from build123d import *

# Parameters (mm, degrees)
F1_DEPTH = 1
F3_DEPTH = 0.05
F4_W     = 3.2
F4_H     = 5
F5_DEPTH = 0.9
F6_R     = 0.25


with BuildPart() as f1:
    # F0 (on Front) → F1 (new body)
    with BuildSketch(Plane.XZ):
        Polygon((0, 0.35), (0, 0), (16, 0), (16, 0.35), (15, 0.35), (15, 1.65), (16, 1.65), (16, 2.35), (15, 2.35), (15, 3.65), (16, 3.65), (16, 4.35), (15, 4.35), (15, 5.65), (16, 5.65), (16, 6.35), (15, 6.35), (15, 7.65), (16, 7.65), (16, 8.35), (15, 8.35), (15, 9.65), (16, 9.65), (16, 10.35), (15, 10.35), (15, 11.65), (16, 11.65), (16, 12.35), (15, 12.35), (15, 13.65), (16, 13.65), (16, 14.35), (15, 14.35), (15, 15.65), (16, 15.65), (16, 16), (0, 16), (0, 15.65), (1, 15.65), (1, 14.35), (0, 14.35), (0, 13.65), (1, 13.65), (1, 12.35), (0, 12.35), (0, 11.65), (1, 11.65), (1, 10.35), (0, 10.35), (0, 9.65), (1, 9.65), (1, 8.35), (0, 8.35), (0, 7.65), (1, 7.65), (1, 6.35), (0, 6.35), (0, 5.65), (1, 5.65), (1, 4.35), (0, 4.35), (0, 3.65), (1, 3.65), (1, 2.35), (0, 2.35), (0, 1.65), (1, 1.65), (1, 0.35), align=None)
        with BuildLine():
            ThreePointArc((0, 13.65), (0.380511, 13), (0, 12.35))
            Line((0, 12.35), (1, 12.35))
            Line((1, 12.35), (1, 13.65))
            Line((1, 13.65), (0, 13.65))
        make_face()
        with BuildLine():
            ThreePointArc((0, 11.65), (0.380511, 11), (0, 10.35))
            Line((0, 10.35), (1, 10.35))
            Line((1, 10.35), (1, 11.65))
            Line((1, 11.65), (0, 11.65))
        make_face()
        with BuildLine():
            ThreePointArc((0, 9.65), (0.380511, 9), (0, 8.35))
            Line((0, 8.35), (1, 8.35))
            Line((1, 8.35), (1, 9.65))
            Line((1, 9.65), (0, 9.65))
        make_face()
        with BuildLine():
            ThreePointArc((0, 7.65), (0.380511, 7), (0, 6.35))
            Line((0, 6.35), (1, 6.35))
            Line((1, 6.35), (1, 7.65))
            Line((1, 7.65), (0, 7.65))
        make_face()
        with BuildLine():
            ThreePointArc((0, 5.65), (0.380511, 5), (0, 4.35))
            Line((0, 4.35), (1, 4.35))
            Line((1, 4.35), (1, 5.65))
            Line((1, 5.65), (0, 5.65))
        make_face()
        with BuildLine():
            ThreePointArc((0, 3.65), (0.380511, 3), (0, 2.35))
            Line((0, 2.35), (1, 2.35))
            Line((1, 2.35), (1, 3.65))
            Line((1, 3.65), (0, 3.65))
        make_face()
        with BuildLine():
            ThreePointArc((0, 1.65), (0.380511, 1), (0, 0.35))
            Line((0, 0.35), (1, 0.35))
            Line((1, 0.35), (1, 1.65))
            Line((1, 1.65), (0, 1.65))
        make_face()
        with BuildLine():
            Line((15, 4.35), (16, 4.35))
            ThreePointArc((16, 4.35), (15.619489, 5), (16, 5.65))
            Line((16, 5.65), (15, 5.65))
            Line((15, 5.65), (15, 4.35))
        make_face()
        with BuildLine():
            Line((15, 6.35), (16, 6.35))
            ThreePointArc((16, 6.35), (15.619489, 7), (16, 7.65))
            Line((16, 7.65), (15, 7.65))
            Line((15, 7.65), (15, 6.35))
        make_face()
        with BuildLine():
            Line((15, 8.35), (16, 8.35))
            ThreePointArc((16, 8.35), (15.619489, 9), (16, 9.65))
            Line((16, 9.65), (15, 9.65))
            Line((15, 9.65), (15, 8.35))
        make_face()
        with BuildLine():
            Line((15, 10.35), (16, 10.35))
            ThreePointArc((16, 10.35), (15.619489, 11), (16, 11.65))
            Line((16, 11.65), (15, 11.65))
            Line((15, 11.65), (15, 10.35))
        make_face()
        with BuildLine():
            Line((15, 12.35), (16, 12.35))
            ThreePointArc((16, 12.35), (15.619489, 13), (16, 13.65))
            Line((16, 13.65), (15, 13.65))
            Line((15, 13.65), (15, 12.35))
        make_face()
        with BuildLine():
            Line((15, 14.35), (16, 14.35))
            ThreePointArc((16, 14.35), (15.619489, 15), (16, 15.65))
            Line((16, 15.65), (15, 15.65))
            Line((15, 15.65), (15, 14.35))
        make_face()
        with BuildLine():
            Line((15, 2.35), (16, 2.35))
            ThreePointArc((16, 2.35), (15.619489, 3), (16, 3.65))
            Line((16, 3.65), (15, 3.65))
            Line((15, 3.65), (15, 2.35))
        make_face()
        with BuildLine():
            Line((15, 0.35), (16, 0.35))
            ThreePointArc((16, 0.35), (15.619489, 1), (16, 1.65))
            Line((16, 1.65), (15, 1.65))
            Line((15, 1.65), (15, 0.35))
        make_face()
        with BuildLine():
            ThreePointArc((0, 15.65), (0.380511, 15), (0, 14.35))
            Line((0, 14.35), (1, 14.35))
            Line((1, 14.35), (1, 15.65))
            Line((1, 15.65), (0, 15.65))
        make_face()
    extrude(amount=F1_DEPTH)

    # F2 (on face) → F3 (join)
    with BuildSketch(Plane.XZ.offset(1)):
        with BuildLine():
            ThreePointArc((16, 14.35), (15.619489, 15), (16, 15.65))
            Line((16, 15.65), (15, 15.65))
            Line((15, 15.65), (15, 14.35))
            Line((15, 14.35), (16, 14.35))
        make_face()
        with BuildLine():
            ThreePointArc((16, 12.35), (15.619493, 12.997842), (15.996242, 13.647876))
            Line((15.996242, 13.647876), (15, 13.647876))
            Line((15, 13.647876), (15, 12.347876))
            Line((15, 12.347876), (16, 12.347876))
            Line((16, 12.347876), (16, 12.35))
        make_face()
        with BuildLine():
            ThreePointArc((16, 10.35), (15.619502, 10.995706), (15.992535, 11.645752))
            Line((15.992535, 11.645752), (15, 11.645752))
            Line((15, 11.645752), (15, 10.345752))
            Line((15, 10.345752), (16, 10.345752))
            Line((16, 10.345752), (16, 10.35))
        make_face()
        with BuildLine():
            ThreePointArc((16, 8.35), (15.619517, 8.99359), (15.988876, 9.643628))
            Line((15.988876, 9.643628), (15, 9.643628))
            Line((15, 9.643628), (15, 8.343628))
            Line((15, 8.343628), (16, 8.343628))
            Line((16, 8.343628), (16, 8.35))
        make_face()
        with BuildLine():
            ThreePointArc((16, 6.35), (15.619538, 6.991495), (15.985264, 7.641505))
            Line((15.985264, 7.641505), (15, 7.641505))
            Line((15, 7.641505), (15, 6.341505))
            Line((15, 6.341505), (16, 6.341505))
            Line((16, 6.341505), (16, 6.35))
        make_face()
        with BuildLine():
            ThreePointArc((16, 4.35), (15.619565, 4.98942), (15.981698, 5.639381))
            Line((15.981698, 5.639381), (15, 5.639381))
            Line((15, 5.639381), (15, 4.339381))
            Line((15, 4.339381), (16, 4.339381))
            Line((16, 4.339381), (16, 4.35))
        make_face()
        with BuildLine():
            ThreePointArc((16, 2.35), (15.619597, 2.987364), (15.978177, 3.637257))
            Line((15.978177, 3.637257), (15, 3.637257))
            Line((15, 3.637257), (15, 2.337257))
            Line((15, 2.337257), (16, 2.337257))
            Line((16, 2.337257), (16, 2.35))
        make_face()
        with BuildLine():
            ThreePointArc((16, 0.35), (15.619634, 0.985327), (15.974699, 1.635133))
            Line((15.974699, 1.635133), (15, 1.635133))
            Line((15, 1.635133), (15, 0.335133))
            Line((15, 0.335133), (16, 0.335133))
            Line((16, 0.335133), (16, 0.35))
        make_face()
        with BuildLine():
            Line((1, 1.635133), (0.025301, 1.635133))
            ThreePointArc((0.025301, 1.635133), (0.380366, 0.985327), (0, 0.35))
            Line((0, 0.35), (0, 0.335133))
            Line((0, 0.335133), (1, 0.335133))
            Line((1, 0.335133), (1, 1.635133))
        make_face()
        with BuildLine():
            Line((1, 3.637257), (0.021823, 3.637257))
            ThreePointArc((0.021823, 3.637257), (0.380403, 2.987364), (0, 2.35))
            Line((0, 2.35), (0, 2.337257))
            Line((0, 2.337257), (1, 2.337257))
            Line((1, 2.337257), (1, 3.637257))
        make_face()
        with BuildLine():
            Line((1, 5.639381), (0.018302, 5.639381))
            ThreePointArc((0.018302, 5.639381), (0.380435, 4.98942), (0, 4.35))
            Line((0, 4.35), (0, 4.339381))
            Line((0, 4.339381), (1, 4.339381))
            Line((1, 4.339381), (1, 5.639381))
        make_face()
        with BuildLine():
            Line((1, 7.641505), (0.014736, 7.641505))
            ThreePointArc((0.014736, 7.641505), (0.380462, 6.991495), (0, 6.35))
            Line((0, 6.35), (0, 6.341505))
            Line((0, 6.341505), (1, 6.341505))
            Line((1, 6.341505), (1, 7.641505))
        make_face()
        with BuildLine():
            Line((1, 9.643628), (0.011124, 9.643628))
            ThreePointArc((0.011124, 9.643628), (0.380483, 8.99359), (0, 8.35))
            Line((0, 8.35), (0, 8.343628))
            Line((0, 8.343628), (1, 8.343628))
            Line((1, 8.343628), (1, 9.643628))
        make_face()
        with BuildLine():
            Line((1, 11.645752), (0.007465, 11.645752))
            ThreePointArc((0.007465, 11.645752), (0.380498, 10.995706), (0, 10.35))
            Line((0, 10.35), (0, 10.345752))
            Line((0, 10.345752), (1, 10.345752))
            Line((1, 10.345752), (1, 11.645752))
        make_face()
        with BuildLine():
            Line((1, 13.647876), (0.003758, 13.647876))
            ThreePointArc((0.003758, 13.647876), (0.380507, 12.997842), (0, 12.35))
            Line((0, 12.35), (0, 12.347876))
            Line((0, 12.347876), (1, 12.347876))
            Line((1, 12.347876), (1, 13.647876))
        make_face()
        with BuildLine():
            Line((1, 15.65), (0, 15.65))
            ThreePointArc((0, 15.65), (0.380511, 15), (0, 14.35))
            Line((0, 14.35), (1, 14.35))
            Line((1, 14.35), (1, 15.65))
        make_face()
    extrude(amount=F3_DEPTH)

    # F4 (on face) → F5 (join)
    with BuildSketch(Plane.XZ.offset(1)):
        with Locations((11.804315, 7.033254)):
            Rectangle(F4_W, F4_H)
    extrude(amount=F5_DEPTH)

    # F6
    f6_edges = [f1.edges().sort_by_distance(p)[0] for p in [
        (10.204315, -1.45, 4.533254),
        (13.404315, -1.45, 4.533254),
        (10.204315, -1.45, 9.533254),
        (13.404315, -1.45, 9.533254),
    ]]
    fillet(f6_edges, radius=F6_R)


solid = f1.part
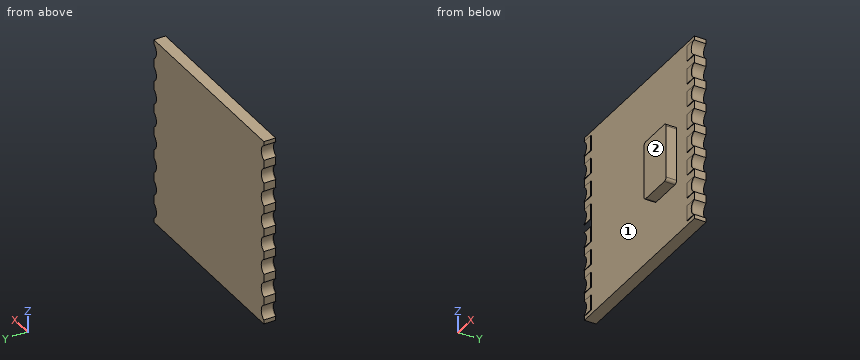
Design review of the part built by this model. Coordinates are the model's own, in mm. Face numbers are marked on the shaded views. Round coordinates to 2 decimals unless told otherwise and drop trailing zeros. Write each loop counter-clockwise with the first axis right and the second up, starting at its lowest first coordinate (ties: lowest second). Pieces come first, ordered by that corner, then holes. Notation, with made-up numbers: (89.25, 73) -> (125.25, 73) arc R15 cw to (125.25, 88) -> close; hole circle Ø3 at (6.25, -39.5). An arc over 180 degrees is marked (long way). One line per item, written item: value. Start each with the question number.
Q1. Add section C-C (z = 13). Give the boundary of the cut face in (x, y).
Q2. Add section D-D (x = 4.75). Give the boundary of the cut face in (y, z).
Q3. Add section A-A (y = -1.25). Give the boundary of the cut face in (x, z), then the cut area to 3 significant figures.
Q4. The part is to be moulded in two halves that separate along X. For the marked faces 1 and 2, say which applies: pulls with the +X half, pulls with the -X half, needs draft (parallel to the pull), parting line crosses it, or undercut.
Q5. Insertion check: P1, Ø0.7, axis at y = -1.5, z = 8, coming from the -X side; P2, Ø0.5, axis at x = 15.5, z = 15.5, coming from the -Y side. Each pin has a flat end and moves straight along its axis. Give the tip position at first contact, or say it passes through.
Q6. Add section B-B (x = 12). Give the boundary of the cut face in (y, z).
Q7. To check wall thickness, follow probe 1 along Y at (x, z) = (13.5, 12.75); probe 2 along X at (y, z) = (-0.55, 3); probe 3 along X at (y, z) = (-1.6, 5.75). State the ranges of each line that lie inside material, in increasing order.
Response:
1. outline: (0.38, -1.05) -> (1, -1.05) -> (1, -1) -> (15, -1) -> (15, -1.05) -> (15.62, -1.05) -> (15.62, 0) -> (0.38, 0) -> close
2. outline: (-1, 0) -> (0, 0) -> (0, 16) -> (-1, 16) -> close
3. outline: (10.2, 4.78) arc R0.25 ccw to (10.45, 4.53) -> (13.15, 4.53) arc R0.25 ccw to (13.4, 4.78) -> (13.4, 9.28) arc R0.25 ccw to (13.15, 9.53) -> (10.45, 9.53) arc R0.25 ccw to (10.2, 9.28) -> close
3. area: 15.9 mm^2
4. face 1: undercut
4. face 2: needs draft
5. P1: stops at x = 10.2
5. P2: stops at y = -1.05
6. outline: (-1.9, 4.53) -> (-1, 4.53) -> (-1, 0) -> (0, 0) -> (0, 16) -> (-1, 16) -> (-1, 9.53) -> (-1.9, 9.53) -> close
7. probe 1: y = -1 to 0
7. probe 2: x = 0.38 to 15.62
7. probe 3: x = 10.2 to 13.4
